Input: part model. Units: mm. Frame: model coordinates. Face numbers are marked on the shaded views. A direction names the side the tool comes from. Round coordinates to 2 decimals unless told otherwise and drop trailing zeros. Order: outer loops, then holes, each group sorted by start corner. A loop starts at its lowest first (then second) coordinate and runs counter-clockwise, first axis right, second up.
Item 1: Mould query, pull axis Z, two halves, no side actions, for the marked faces 3, 4 and 5. Classes: released by +Z, released by -Z, zero draft, split by the parting line, or undercut.
Item 2: Reachability of the marked faces 1 and 2 from +Z, -Z, +X, -X, +Y, -Y: full face, straight path, thin tool, end or side. Return the list, or none.
Item 3: Line query: L1, parallel to X at y = 1.8, z = -11.6 (3 decimals); L2, parallel to Y at x = 35, z = -9; L3, parallel to Z at x = 27, y = 7.75. Output: solid intervals per line, ascending.
Item 4: Cut plane B-B on z = -7. Output: boundary loops of the cut face in (x, y), then the cut area to 3 significant figures.
Item 5: Cut plane A-A on y = 10. Output: boundary loops of the cut face in (x, z), then the cut area to 3 significant figures.
Item 6: Cut plane C-C on x = -15. Output: boundary loops of the cut face in (y, z), then the cut area to 3 significant figures.
Item 7: Cut plane D-D on y = 14. Output: boundary loops of the cut face in (x, z).
Item 8: First-contact query: pin 1 (1.5 mm diameter, centred on x = -19, z = 10.5, fed in from +Y); pin 2 (10 mm diameter, centred on y = 10.5, z = -11, fed in from -X); pin 3 (3 mm diameter, centred on y = 11.5, z = -12, fed in from +X); pin 4 (2 mm diameter, centred on x = -41.305, z = -11.6, fed in from -Y) (3 decimals). Flat tips, straight axial feed; report the tip coordinate or a pass-through.
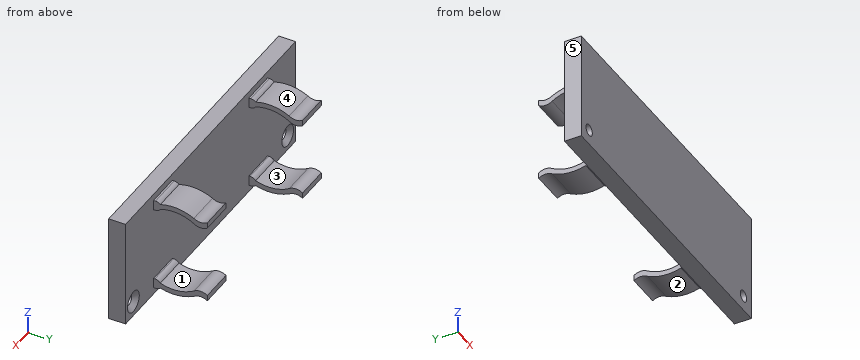
Autodesk Inventor part; units mm, degrees
ref_plane "YZ Plane" through (0, 0, 0) normal (1, 0, 0) x (0, 1, 0)
ref_plane "XZ Plane" through (0, 0, 0) normal (0, 1, 0) x (-1, 0, 0)
ref_plane "XY Plane" through (0, 0, 0) normal (0, 0, 1) x (1, 0, 0)
sketch "Sketch1" plane through (0, 0, 0) normal (0, 1, 0) x (-1, 0, 0)
  line L0 (41.305, -11.6) -> (-41.305, -11.6) construction
  line L1 (0, 107.889) -> (0, -128.889) construction
  line L2 (45.5, -16.1) -> (-45.5, -16.1)
  line L3 (-45.5, -16.1) -> (-45.5, 16.1)
  line L4 (-45.5, 16.1) -> (45.5, 16.1)
  line L5 (45.5, 16.1) -> (45.5, -16.1)
  line L6 (62.4324, 0) -> (-80.3334, 0) construction
  point P0 (0, 0)
  point P1 (45.5, 0)
  point P2 (0, 16.1)
  point P3 (0, -11.6)
  dimension "d1" = 82.61
  dimension "d2" = 91
  dimension "d3" = 32.2
  dimension "d4" = 4.5
extrude "Extrusion1" add sketch "Sketch1" along normal blind 5
sketch "Sketch2" plane through (0, 5, 0) normal (0, 1, 0) x (1, 0, 0)
  line L0 (-45.5, -16.1) -> (45.5, -16.1)
  line L1 (45.5, -16.1) -> (45.5, 16.1)
  line L2 (45.5, 16.1) -> (-45.5, 16.1)
  line L3 (-45.5, 16.1) -> (-45.5, -16.1)
  point P0 (0, 0)
  point P1 (41.305, 11.6)
  point P2 (-41.305, 11.6)
  point P3 (41.305, 11.6)
  point P4 (-41.305, 11.6)
hole "Hole1" at (41.305, 5, -11.6) at (-41.305, 5, -11.6) direction (0, -1, 0) diameter 3.4 depth 5 countersink diameter 6.3 countersink angle 90
ref_plane "Work Plane1" through (25.5, 0, 16.1) normal (1, 0, 0) x (0, 0, -1)
ref_plane "Work Plane2" through (0, 0, 16.1) normal (1, 0, 0) x (0, 0, -1)
sketch "Sketch3" plane through (25.5, 0, 16.1) normal (1, 0, 0) x (0, 0, -1)
  line L0 (0, 5) -> (32.2, 5)
  line L1 (2, 5) -> (5, 5)
  line L2 (5, 5) -> (5, 7)
  line L3 (5, 7) -> (4.18, 7)
  line L4 (2, 7) -> (2, 5)
  line L5 (16.1, 17.288) -> (16.1, -5.2059) construction
  line L6 (0, 0) -> (0, 5) construction
  arc A0 (3.4943, 16.9472) -> (3.4943, 20.9472) centre (0.622, 18.9472) ccw
  arc A1 (5.2405, 16.979) -> (5.2223, 20.9472) centre (2.3482, 18.9499) ccw
  line L7 (3.4943, 20.9472) -> (5.2223, 20.9472)
  arc A2 (3.4943, 16.9472) -> (2.5975, 7) centre (15, 10.896) ccw
  arc A3 (5.2405, 16.979) -> (4.18, 7) centre (15, 10.896) ccw
  line L8 (2.5975, 7) -> (2, 7)
  line L9 (27.2, 5) -> (27.2, 7)
  line L10 (27.2, 7) -> (28.02, 7)
  line L11 (30.2, 7) -> (30.2, 5)
  line L12 (28.7057, 5) -> (28.7057, 18.917) construction
  arc A4 (28.7057, 20.9472) -> (28.7057, 16.9472) centre (31.578, 18.9472) ccw
  arc A5 (26.9777, 20.9472) -> (26.9595, 16.979) centre (29.8518, 18.9499) ccw
  line L13 (28.7057, 20.9472) -> (26.9777, 20.9472)
  arc A6 (29.6025, 7) -> (28.7057, 16.9472) centre (17.2, 10.896) ccw
  arc A7 (28.02, 7) -> (26.9595, 16.979) centre (17.2, 10.896) ccw
  line L14 (29.6025, 7) -> (30.2, 7)
  point P0 (16.1, 0)
  dimension "d20" = 3
  dimension "d21" = 2
  dimension "d23" = 2
  dimension "d25" = 4
  dimension "d26" = 3.5
  dimension "d27" = 3.5
  dimension "d31" = 16.1
  dimension "d32" = 1.5
  dimension "d33" = 0.5975
  dimension "d34" = 13
extrude "Extrusion2" add sketch "Sketch3" along normal mid plane 10
mirror "Mirror1" about plane through (0, 0, 16.1) normal (1, 0, 0) of "Extrusion2"
fillet "Fillet1" radius 2 8 edges at (25.5, 7, 14.1) (25.5, 7, 11.1) (-25.5, 7, 14.1) (-25.5, 7, 11.1) (25.5, 7, -11.1) (25.5, 7, -14.1) (-25.5, 7, -14.1) (-25.5, 7, -11.1)
properties part number "powerbank_mount_3DPrint"
From the geometry:
1. face 3: undercut
1. face 4: released by +Z
1. face 5: zero draft
2. face 1: +X, -X
2. face 2: -Z, +X, -X
3. L1: x = -45.5 to -43.005, -39.605 to 39.605, 43.005 to 45.5
3. L2: y = 0 to 5
3. L3: z = -13.71 to -12.16, 12.16 to 13.71
4. outline: (-45.5, 0) - (45.5, 0) - (45.5, 5) - (-45.5, 5) - close
4. area: 455 mm2
5. outline: (-30.5, -14.07) - (-20.5, -14.07) - (-20.5, -12.57) - (-30.5, -12.57) - close; (-30.5, 12.57) - (-20.5, 12.57) - (-20.5, 14.07) - (-30.5, 14.07) - close; (20.5, -14.07) - (30.5, -14.07) - (30.5, -12.57) - (20.5, -12.57) - close; (20.5, 12.57) - (30.5, 12.57) - (30.5, 14.07) - (20.5, 14.07) - close
5. area: 60.2 mm2
6. outline: (0, -16.1) - (5, -16.1) - (5, 16.1) - (0, 16.1) - close
6. area: 161 mm2
7. outline: (-30.5, -13.72) - (-20.5, -13.72) - (-20.5, -12.17) - (-30.5, -12.17) - close; (-30.5, 12.17) - (-20.5, 12.17) - (-20.5, 13.72) - (-30.5, 13.72) - close; (20.5, -13.72) - (30.5, -13.72) - (30.5, -12.17) - (20.5, -12.17) - close; (20.5, 12.17) - (30.5, 12.17) - (30.5, 13.72) - (20.5, 13.72) - close
8. pin 1: stops at y = 5
8. pin 2: stops at x = -30.5
8. pin 3: stops at x = 30.5
8. pin 4: passes through
